Autodesk Inventor part; units mm, degrees
ref_plane "YZ Plane" through (0, 0, 0) normal (1, 0, 0) x (0, 1, 0)
ref_plane "XZ Plane" through (0, 0, 0) normal (0, 1, 0) x (-1, 0, 0)
ref_plane "XY Plane" through (0, 0, 0) normal (0, 0, 1) x (1, 0, 0)
sketch "Sketch1" plane through (0, 0, 0) normal (1, 0, 0) x (0, 1, 0)
  circle A0 centre (0, 0) radius 0.45
  dimension "d0" = 0.9
sketch "Sketch2" plane through (0, 0, 0) normal (0, 1, 0) x (-1, 0, 0)
  line L0 (0, 0) -> (0.1, 0)
  line L1 (0.1, 0) -> (78.0289, 0)
  line L2 (81.5645, 1.4645) -> (84.9995, 4.8995)
  line L3 (88.535, 6.364) -> (116.464, 6.364)
  arc A0 (88.535, 6.364) -> (84.9995, 4.8995) centre (88.535, 1.364) ccw
  arc A1 (78.0289, 0) -> (81.5645, 1.4645) centre (78.0289, 5) ccw
  point P0 (80.1, 0)
  point P1 (86.464, 6.364)
  dimension "d1" = 0.1
  dimension "d4" = 80
  dimension "d6" = 9
  dimension "d7" = 30
  dimension "d8" = 5
sweep "Sweep2" add profiles "Sketch1" path "Sketch2"
properties part number "cable medio"
CAD build for the part. Positions are in the model's coordinates, mm. Round coordinates to 2 decimals unless told otherwise and drop trailing zeros. Loops run counter-clockwise (first coordinate to the right, second up) from the corner with the lowest first, then second, coordinate; pieces in that order, holes last. Notation, with made-up numbers: M -39.75,-6 L -17.75,-6 A20 cw -17.75,10 Z; hole C -9.75,11 d11. An arc over 180 degrees is marked long. Return JSON: item names as keys, results as strings. Group by question number.
(1) Saw through at A-A, the plane x = -28. List the corners of the cut face in (y, z).
(2) Drop a flat-ended pin along its axis: P1, Ø1.5, axis at x = -91.5, z = 5, coming from the +Y side. Give the stop position or say it passes through.
(3) Wall check: probe 1 along Z at (x, y) = (-57.5, -0.1); probe 2 along Z at (x, y) = (-108.5, -0.05); probe 3 along X at (y, z) = (-0.05, 4.25). Give the ranges that are in metal, low to high. Write a range as [from, to].
Answer list:
{
 "1": {"outline": "C 0,0 d0.9"},
 "2": {"P1": "through"},
 "3": {"probe 1": "[-0.44, 0.44]", "probe 2": "[5.92, 6.81]", "probe 3": "[-84.98, -83.72]"}
}
